Could you check a few things on this model? Use its own coordinates, in mm. A direction names the side the tool comes from. Coordinates: 2 decimals unless noted, no trailing zeros. Order: outer loops, then holes, each group sorted by start corner. A loop starts at its lowest first (then second) coordinate and runs counter-clockwise, first axis right, second up. Notation, with made-up numbers: (41, 50) -> (50, 50) arc R8 ccw to (50, 63) -> close; hole circle Ø8 at (57, 83.25). An arc over 180 degrees is marked (long way). Put each result on its own line as item: value. Start each with the question number.
Q1. Please list where these lines run through material, in increasing order: line 1 along Y through (x, z) = (24, 20); line 2 along Y through (x, z) = (33, 10.5); line 3 along Z through (x, y) = (22, 4).
Q2. For faces 1 (the face through (32, 0, -3)), 2 (the face through (20.96, 3.16, 3.01)), 3 (the face through (31.25, 3.16, -3.03)), 4 (the face through (31.3, 3.16, 2.94)), 5 (the face through (20.91, 3.16, -2.94)), which set-ups out of +Z, -Z, +X, -X, +Y, -Y let a thin tool reach every point of the face, with its end or its side?
Q3. Will these pins go through, and if not, where does the flat tip stop? pin 1 (1.9 mm diameter, centred on x = 25, y = 3, fed in from -Z); pin 2 (5 mm diameter, centred on y = 9, z = -0.5, fed in from -X); pin 3 (2 mm diameter, centred on x = 41, y = -9.5, fed in from +Z); pin 4 (10 mm diameter, centred on x = 39.5, y = 11.5, fed in from -Z).
Q4. If we section it at A-A (y = 1): Please give me the cut outline in (x, z), and give its area (3 significant figures).
Q5. If we section it at B-B (y = 12): Please give me the cut outline in (x, z) (1 decimal), and give its area (3 significant figures).
Q6. If we section it at C-C (y = -5): Please give me the cut outline in (x, z).
from build123d import *

# Parameters (mm, degrees)
SKETCH2_OUTSIDE_W  = 67.698
SKETCH2_OUTSIDE_H  = 67.698
CUT_EXTRUDE1_DEPTH = 6.223


with BuildPart() as part:
    # Sketch1 → Revolve1 (revolve)
    with BuildSketch(Plane.XY, mode=Mode.PRIVATE) as revolve1_sk:
        with BuildLine():
            Line((9.373695388, -16.129), (26.106953114, -16.129))
            Line((26.106953114, -16.129), (26.106953114, 20.955))
            Line((26.106953114, 20.955), (22.868453114, 20.955))
            Line((22.868453114, 20.955), (21.344453114, 19.431))
            Line((21.344453114, 19.431), (21.344453114, 6.223))
            Line((21.344453114, 6.223), (19.214545601, 6.223))
            Line((19.214545601, 6.223), (19.214545601, 0))
            Line((19.214545601, 0), (18.525304849, 0))
            Line((18.525304849, 0), (18.525304849, -1.524))
            Line((18.525304849, -1.524), (5.532953114, -1.524))
            ThreePointArc((5.532953114, -1.524), (2.479666033, -2.788712919), (1.214953114, -5.842))
            Line((1.214953114, -5.842), (1.214953114, -7.0612))
            ThreePointArc((1.214953114, -7.0612), (2.479666033, -10.114487081), (5.532953114, -11.3792))
            Line((5.532953114, -11.3792), (7.341695388, -11.3792))
            Line((7.341695388, -11.3792), (7.341695388, -14.097))
            ThreePointArc((7.341695388, -14.097), (7.936854408, -15.533840979), (9.373695388, -16.129))
        make_face()
    revolve(revolve1_sk.sketch.rotate(Axis((26.106953114, 20.955, 0), (0, -1, 0)), 270), axis=Axis((26.106953114, 20.955, 0), (0, -1, 0)))

    # Sketch2 outside → Cut-Extrude1 (cut)
    with BuildSketch(Plane(origin=(0, 6.223, 0), x_dir=(1, 0, 0), z_dir=(0, 1, 0))):
        with Locations((26.107, 0)):
            Rectangle(SKETCH2_OUTSIDE_W, SKETCH2_OUTSIDE_H)
        Polygon((22.660749357, 5.969), (29.553156871, 5.969), (32.999360628, 0), (29.553156871, -5.969), (22.660749357, -5.938392769), (19.214545601, 0), align=None, mode=Mode.SUBTRACT)
    extrude(amount=-CUT_EXTRUDE1_DEPTH, mode=Mode.SUBTRACT)


solid = part.part
The answers:
1. line 1: -11.38 to -1.52
1. line 2: -16.13 to -1.52
1. line 3: -4.82 to 4.8
2. face 1: +Y
2. face 2: +Z, -X, +Y
2. face 3: -Z, +X, +Y
2. face 4: +Z, +X, +Y
2. face 5: -Z, -X, +Y
3. pin 1: z = -5.97
3. pin 2: x = 21.34
3. pin 3: z = 20.02
3. pin 4: through
4. outline: (19.21, 0) -> (22.66, -5.97) -> (29.55, -5.97) -> (33, 0) -> (29.55, 5.97) -> (22.66, 5.94) -> close
4. area: 123 mm^2
5. outline: circle Ø9.5 at (26.1, 0)
5. area: 71.3 mm^2
6. outline: circle Ø49.62 at (26.11, 0)
